Part print with two shaded views. Sizes in mm from the minimum x, y, z corner. A direction names the side the tool comes from. Round coordinates to 2 decimals unless told otherwise and drop trailing zeros. Write each loop counter-clockwise with the first axis right and the second up, starting at its lowest first coordinate (ties: lowest second). Pieces come first, ordered by that corner, then holes. Notation, with made-up numbers: (-22, 83) -> (6, 83) arc R12 ccw to (6, 102) -> close; hole circle Ø3 at (-5, -17). An arc over 180 degrees is marked (long way). Answer in a Markdown table with one row per item.
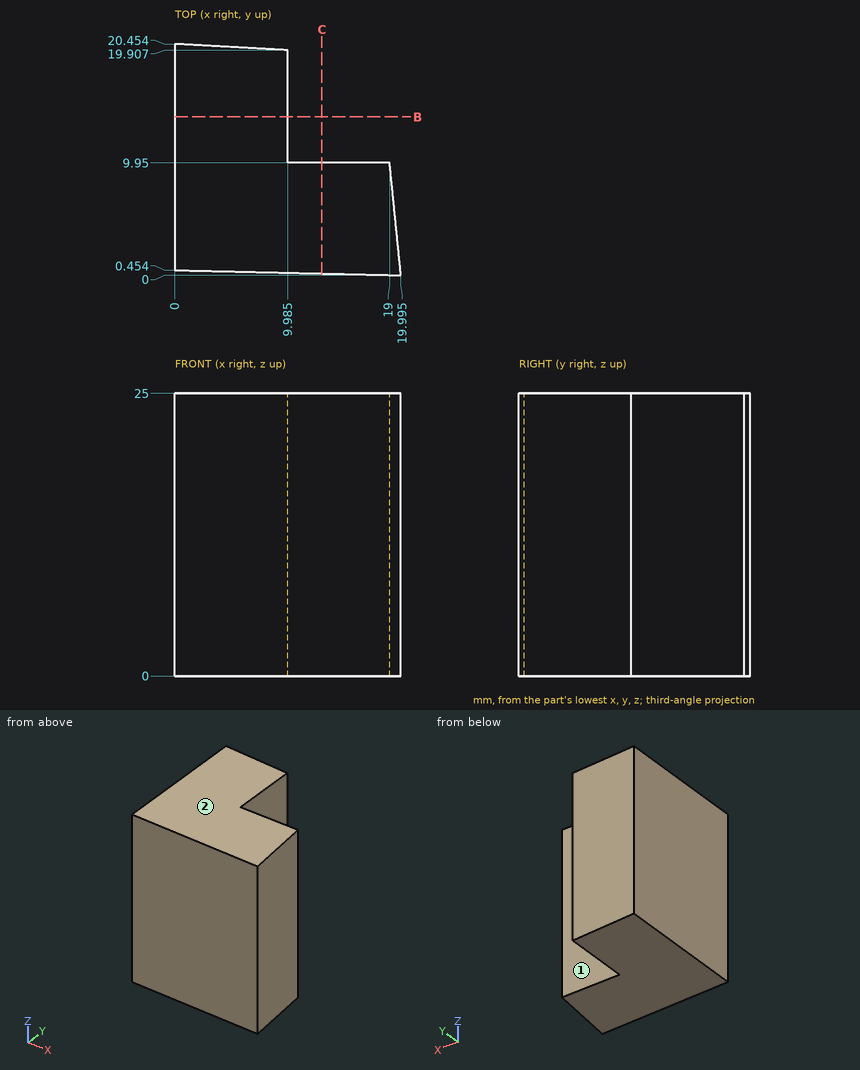
Q1. Saw through at C-C on x = 13. Write the cut outline in (y, z).
A:
| item | result |
|---|---|
| outline | (0.16, 0) -> (9.95, 0) -> (9.95, 25) -> (0.16, 25) -> close |
Q2. Which spindle directions (+Z, -Z, +X, -X, +Y, -Y) get a long thin tool onto all of the face, cutting with end or side? Do the marked faces 1 and 2. Say none if no direction does.
A:
| item | result |
|---|---|
| face 1 | +Z, -Z, +X, +Y |
| face 2 | +Z, +X, -X, +Y, -Y |
Q3. Wall check: line 1 (X direction, y = 11, z = 23.5) (1 decimal); line 2 (Y direction, x = 4.75, z = 9) (1 decimal); line 3 (Y direction, x = 7, z = 17) (1 decimal). Give the ranges that are in metal, low to high. Write a range as [from, to].
A:
| item | result |
|---|---|
| line 1 | [0, 10] |
| line 2 | [0.3, 20.2] |
| line 3 | [0.3, 20.1] |
Q4. Saw through at B-B on y = 14. Write the cut outline in (x, z) (1 decimal).
A:
| item | result |
|---|---|
| outline | (0, 0) -> (10, 0) -> (10, 25) -> (0, 25) -> close |
Q5. Drop flat-ended pins along their axis: P1, Ø5, axis at x = 6.5, y = 13, coming from the -Z side; P2, Ø11, axis at y = 15, z = 17.5, coming from the +X side (1 decimal); P3, Ø5, axis at x = 3, z = 8, coming from the +Y side; P4, Ø1.5, axis at x = 15, z = 11.5, coming from the +Y side. Give the stop position or say it passes through.
A:
| item | result |
|---|---|
| P1 | z = 0 |
| P2 | x = 19 |
| P3 | y = 20.43 |
| P4 | y = 9.95 |
